from build123d import *

# Parameters (mm, degrees)
SKETCH1_R      = 1.4
SHAPE_DEPTH    = 4
SKETCH2_R      = 1
NUT_CUTS_DEPTH = 2


with BuildPart() as part:
    # Sketch1 → Shape (new body)
    with BuildSketch(Plane.XY):
        with BuildLine():
            Line((74.415384615, 55.186207026), (78.5, 50.928752721))
            ThreePointArc((78.5, 50.928752721), (78.788582233, 78.788582233), (50.928752721, 78.5))
            Line((50.928752721, 78.5), (55.186207026, 74.415384615))
            ThreePointArc((55.186207026, 74.415384615), (70.07407211, 77.617994778), (78.6, 65))
            ThreePointArc((78.6, 65), (77.51018047, 59.665641124), (74.415384615, 55.186207026))
        make_face()
        with Locations((79.925281419, 57.965373175)):
            Circle(SKETCH1_R, mode=Mode.SUBTRACT)
        with Locations((57.965373175, 79.925281419)):
            Circle(SKETCH1_R, mode=Mode.SUBTRACT)
        with Locations((76.66726189, 76.66726189)):
            Circle(SKETCH1_R, mode=Mode.SUBTRACT)
    extrude(amount=SHAPE_DEPTH)

    # Sketch2 → Nut cuts (cut)
    with BuildSketch(Plane.XY):
        with Locations((56.258688641, 79.120881926)):
            Circle(SKETCH2_R)
        with Locations((56.415400513, 81.001113835)):
            Circle(SKETCH2_R)
        with Locations((58.122085046, 81.805513328)):
            Circle(SKETCH2_R)
        with Locations((59.672057709, 80.729680912)):
            Circle(SKETCH2_R)
        with Locations((59.515345837, 78.849449003)):
            Circle(SKETCH2_R)
        with Locations((57.808661304, 78.04504951)):
            Circle(SKETCH2_R)
        Polygon((60.576620219, 81.156021931), (58.205144148, 82.802057951), (55.593897104, 81.571317438), (55.354126131, 78.694540907), (57.725602202, 77.048504887), (60.336849246, 78.2792454), align=None)
    extrude(amount=NUT_CUTS_DEPTH, mode=Mode.SUBTRACT)


solid = part.part
Build history of the part. All positions in model axes, mm. A direction names the side the tool comes from. Give positions to 0.01 mm unless a question says otherwise; leave off trailing zeros. Order: outer loops, then holes, each group sorted by start corner. A loop starts at its lowest first (then second) coordinate and runs counter-clockwise, first axis right, second up. Notation, with made-up numbers: M 2,42 L 47,42 A15 cw 47,59 Z; hole C 21.25,21 d4. An arc over 180 degrees is marked long. Use one line per item in the form item = value.
Q1. Pin check, flat tips, straight feed: P1, Ø1.5, axis at y = 60.5, z = 1.5, coming from the -X side; P2, Ø1.5, axis at x = 77, z = 3.5, coming from the -Y side; P3, Ø1.5, axis at x = 73.5, z = 3, coming from the +Y side. Stop position of each tip, or through.
Conclusion:
P1 = 77.55
P2 = 51.71
P3 = 82.89
Q2. Pull direction X, two halves, no side cores. Call faces 1 (the cylindrical face through (60.6, 81.1, 1)), 2 (the flat face through (76.429, 53.087, 1.972)), 3 (the flat face through (75, 75, 4)): released by +X, released by -X, zero draft, split by the parting line, or undercut.
Conclusion:
face_1 = undercut
face_2 = released by -X
face_3 = zero draft
Q3. Which spindle directions (+Z, -Z, +X, -X, +Y, -Y) get a long thin tool onto all of the face, cutting with end or side? Do faces 4 (the flat face through (59.026, 77.661, 0.986)), 5 (the flat face through (53.028, 76.486, 1.972)). Say none if no direction does.
Conclusion:
face_4 = -Z
face_5 = +Z, -Z, -X, -Y
Q4. Slice it at B-B, the plane x = 65. Write the cut outline in (y, z).
Conclusion:
outline = M 78.6,0 L 84.5,0 L 84.5,4 L 78.6,4 Z
Q5. Slice it at C-C, the plane y = 73.5. Write the cut outline in (x, z).
Conclusion:
outline = M 75.62,0 L 82.55,0 L 82.55,4 L 75.62,4 Z
Q6. Wall check: probe 1 along X at (y, z) = (64.5, 3.75); probe 2 along X at (y, z) = (77, 2.6); probe 3 along X at (y, z) = (75.5, 1.9). Give the ranges that are in metal, low to high.
Conclusion:
probe_1 = 78.59 to 84.49
probe_2 = 52.49 to 58.6, 71.4 to 75.31, 78.03 to 80.37
probe_3 = 54.06 to 56.36, 73.64 to 75.89, 77.44 to 81.43
Q7. Slice it at A-A, the plane z = 1.4. Write the cut outline in (x, y).
Conclusion:
outline = M 50.93,78.5 L 55.19,74.42 A13.6 cw long 74.42,55.19 L 78.5,50.93 A19.5 ccw long Z; hole M 55.44,79.69 A1 ccw 56.18,78.12 L 56.9,77.62 A1 ccw 58.63,77.47 L 59.43,77.85 A1 ccw 60.42,79.28 L 60.49,80.16 A1 ccw 59.76,81.73 L 59.03,82.23 A1 ccw 57.3,82.38 L 56.5,82 A1 ccw 55.51,80.57 Z; hole C 76.67,76.67 d2.8; hole C 79.93,57.97 d2.8
